from build123d import *

# Parameters (mm, degrees)
SKETCH_4_R          = 1.5
CUT_EXTRUDE_1_DEPTH = 20
SKETCH_5_R          = 1.5
CUT_EXTRUDE_2_DEPTH = 65.884590004
SKETCH3_R           = 5
SKETCH3_W           = 30
SKETCH3_H           = 42
CUT_EXTRUDE1_DEPTH  = 65.884590004
CUT_EXTRUDE2_DEPTH  = 42
CUT_EXTRUDE_3_DEPTH = 0.6


with BuildPart() as part:
    # Эскиз1 → Loft 1 section 0
    with BuildSketch(Plane(origin=(0, 0, 0), x_dir=(1, 0, 0), z_dir=(0, 1, 0))):
        with BuildLine():
            Line((-50.1, -40), (50.1, -40))
            Line((50.1, -40), (50.1, 40))
            Line((50.1, 40), (-50.1, 40))
            Line((-50.1, 40), (-50.1, -40))
        make_face()
    # Эскиз2 → Loft 1 section 1
    with BuildSketch(Plane(origin=(0, 10, 0), x_dir=(1, 0, 0), z_dir=(0, 1, 0))):
        with BuildLine():
            Line((40.1, -30), (40.1, 30))
            Line((40.1, 30), (-40.1, 30))
            Line((-40.1, 30), (-40.1, -30))
            Line((-40.1, -30), (40.1, -30))
        make_face()
    loft()

    # Эскиз4 → Вырез-Вытянуть1 (cut)
    with BuildSketch(Plane.XY.offset(40)):
        with Locations((-35.1, 5)):
            Circle(SKETCH_4_R)
        with Locations(Location((35.1, 5, 0), (0, 0, 270))):
            Circle(SKETCH_4_R)
    cut_extrude_1 = extrude(amount=-CUT_EXTRUDE_1_DEPTH, mode=Mode.SUBTRACT)

    # Зеркальное отражение1: Вырез-Вытянуть1 across plane
    add(cut_extrude_1.mirror(Plane.XY), mode=Mode.SUBTRACT)

    # Эскиз5 → Вырез-Вытянуть2 (cut, through all)
    with BuildSketch(Plane.XZ):
        with Locations(Location((-45.1, 15, 0), (0, 0, 270))):
            Circle(SKETCH_5_R)
        with Locations(Location((-45.1, -15, 0), (0, 0, 180))):
            Circle(SKETCH_5_R)
        with Locations(Location((45.1, -15, 0), (0, 0, 270))):
            Circle(SKETCH_5_R)
        with Locations((45.1, 15)):
            Circle(SKETCH_5_R)
    extrude(amount=-CUT_EXTRUDE_2_DEPTH, mode=Mode.SUBTRACT)

    # Cut-Loft1: read off the stored shape, not the designer's step
    # Cut-Loft1: loft between two sections, ruled curve by curve
    cut_loft1_from = [
        Edge.make_bspline([(-43.923484762, 2.8, 15.930490137), (-45.784465036, 2.8, 18.283520613), (-48.137495512, 2.8, 16.422540339), (-46.276515238, 2.8, 14.069509863), (-44.415534964, 2.8, 11.716479387), (-42.062504488, 2.8, 13.577459661), (-43.923484762, 2.8, 15.930490137)], [0, 0, 0, 0, 0.5, 0.5, 0.5, 1, 1, 1, 1], 3, [1, 0.333333333, 0.333333333, 1, 0.333333333, 0.333333333, 1]),
    ]
    cut_loft1_to = [
        Edge.make_bspline([(-43.881334244, 0, 18.066733405), (-50.014801053, 0, 20.504064917), (-52.452132565, 0, 14.370598107), (-46.318665756, 0, 11.933266595), (-40.185198947, 0, 9.495935083), (-37.747867435, 0, 15.629401893), (-43.881334244, 0, 18.066733405)], [0, 0, 0, 0, 0.5, 0.5, 0.5, 1, 1, 1, 1], 3, [1, 0.333333333, 0.333333333, 1, 0.333333333, 0.333333333, 1]),
    ]
    cut_loft1 = Solid(Shell([*[Face.make_surface_from_curves(cut_loft1_from[k], cut_loft1_to[k]) for k in range(1)], Face(Wire(cut_loft1_from)), Face(Wire(cut_loft1_to))]))
    add(cut_loft1, mode=Mode.SUBTRACT)

    # Mirror1: Cut-Loft1 across plane
    add(cut_loft1.mirror(Plane.XY), mode=Mode.SUBTRACT)

    # Mirror2: read off the stored shape, not the designer's step
    # Mirror2: loft between two sections, ruled curve by curve
    mirror2_from = [
        Edge.make_bspline([(43.923484762, 2.8, 15.930490137), (45.784465036, 2.8, 18.283520613), (48.137495512, 2.8, 16.422540339), (46.276515238, 2.8, 14.069509863), (44.415534964, 2.8, 11.716479387), (42.062504488, 2.8, 13.577459661), (43.923484762, 2.8, 15.930490137)], [0, 0, 0, 0, 0.5, 0.5, 0.5, 1, 1, 1, 1], 3, [1, 0.333333333, 0.333333333, 1, 0.333333333, 0.333333333, 1]),
    ]
    mirror2_to = [
        Edge.make_bspline([(43.881334244, 0, 18.066733405), (50.014801053, 0, 20.504064917), (52.452132565, 0, 14.370598107), (46.318665756, 0, 11.933266595), (40.185198947, 0, 9.495935083), (37.747867435, 0, 15.629401893), (43.881334244, 0, 18.066733405)], [0, 0, 0, 0, 0.5, 0.5, 0.5, 1, 1, 1, 1], 3, [1, 0.333333333, 0.333333333, 1, 0.333333333, 0.333333333, 1]),
    ]
    mirror2 = Solid(Shell([*[Face.make_surface_from_curves(mirror2_from[k], mirror2_to[k]) for k in range(1)], Face(Wire(mirror2_from)), Face(Wire(mirror2_to))]))
    add(mirror2, mode=Mode.SUBTRACT)

    # Mirror2 2: loft between two sections, ruled curve by curve
    mirror2_2_from = [
        Edge.make_bspline([(43.923484762, 2.8, -15.930490137), (45.784465036, 2.8, -18.283520613), (48.137495512, 2.8, -16.422540339), (46.276515238, 2.8, -14.069509863), (44.415534964, 2.8, -11.716479387), (42.062504488, 2.8, -13.577459661), (43.923484762, 2.8, -15.930490137)], [0, 0, 0, 0, 0.5, 0.5, 0.5, 1, 1, 1, 1], 3, [1, 0.333333333, 0.333333333, 1, 0.333333333, 0.333333333, 1]),
    ]
    mirror2_2_to = [
        Edge.make_bspline([(43.881334244, 0, -18.066733405), (50.014801053, 0, -20.504064917), (52.452132565, 0, -14.370598107), (46.318665756, 0, -11.933266595), (40.185198947, 0, -9.495935083), (37.747867435, 0, -15.629401893), (43.881334244, 0, -18.066733405)], [0, 0, 0, 0, 0.5, 0.5, 0.5, 1, 1, 1, 1], 3, [1, 0.333333333, 0.333333333, 1, 0.333333333, 0.333333333, 1]),
    ]
    mirror2_2 = Solid(Shell([*[Face.make_surface_from_curves(mirror2_2_from[k], mirror2_2_to[k]) for k in range(1)], Face(Wire(mirror2_2_from)), Face(Wire(mirror2_2_to))]))
    add(mirror2_2, mode=Mode.SUBTRACT)

    # Sketch3 → Cut-Extrude1 (cut, through all)
    with BuildSketch(Plane.XZ):
        with Locations(Location((-25, -12, 0), (0, 0, 270))):
            Circle(SKETCH3_R)
        with Locations((0, 2)):
            Rectangle(SKETCH3_W, SKETCH3_H)
    extrude(amount=-CUT_EXTRUDE1_DEPTH, mode=Mode.SUBTRACT)

    # Sketch4 → Cut-Extrude2 (cut)
    with BuildSketch(Plane.XY.offset(-19)):
        Polygon((-15, 8.8), (-17, 6.8), (-15, 4.8), align=None)
        Polygon((15, 4.8), (15, 8.8), (17, 6.8), align=None)
    extrude(amount=CUT_EXTRUDE2_DEPTH, mode=Mode.SUBTRACT)

    # Loft 1 2: read off the stored shape, not the designer's step
    # Loft 1 2: loft between two sections, ruled curve by curve
    loft_1_2_from = [
        Edge.make_bspline([(-23, 6.8, -18.708203932), (-14.818181818, 6.8, -16.268857048), (-14.818181818, 6.8, -7.731142952), (-23, 6.8, -5.291796068)], [0, 0, 0, 0, 1, 1, 1, 1], 3, [1, 0.523809524, 0.523809524, 1]),
        Edge.make_line((-23, 6.8, -5.291796068), (-23, 6.8, -18.708203932)),
    ]
    loft_1_2_to = [
        Edge.make_bspline([(-23, 4.8, -16.582575695), (-18.333333333, 4.8, -14.545875386), (-18.333333333, 4.8, -9.454124614), (-23, 4.8, -7.417424305)], [0, 0, 0, 0, 1, 1, 1, 1], 3, [1, 0.6, 0.6, 1]),
        Edge.make_line((-23, 4.8, -7.417424305), (-23, 4.8, -16.582575695)),
    ]
    loft_1_2 = Solid(Shell([*[Face.make_surface_from_curves(loft_1_2_from[k], loft_1_2_to[k]) for k in range(2)], Face(Wire(loft_1_2_from)), Face(Wire(loft_1_2_to))]))
    add(loft_1_2, mode=Mode.SUBTRACT)

    # Вырез-По сечениям2: read off the stored shape, not the designer's step
    # Вырез-По сечениям2: loft between two sections, ruled curve by curve
    loft_2_from = [
        Edge.make_bspline([(-27, 6.8, -5.291796068), (-35.181818182, 6.8, -7.731142952), (-35.181818182, 6.8, -16.268857048), (-27, 6.8, -18.708203932)], [0, 0, 0, 0, 1, 1, 1, 1], 3, [1, 0.523809524, 0.523809524, 1]),
        Edge.make_line((-27, 6.8, -18.708203932), (-27, 6.8, -5.291796068)),
    ]
    loft_2_to = [
        Edge.make_bspline([(-27, 4.8, -7.417424305), (-31.666666667, 4.8, -9.454124614), (-31.666666667, 4.8, -14.545875386), (-27, 4.8, -16.582575695)], [0, 0, 0, 0, 1, 1, 1, 1], 3, [1, 0.6, 0.6, 1]),
        Edge.make_line((-27, 4.8, -16.582575695), (-27, 4.8, -7.417424305)),
    ]
    loft_2 = Solid(Shell([*[Face.make_surface_from_curves(loft_2_from[k], loft_2_to[k]) for k in range(2)], Face(Wire(loft_2_from)), Face(Wire(loft_2_to))]))
    add(loft_2, mode=Mode.SUBTRACT)

    # Зеркальное отражение2: Loft 1 2, Вырез-По сечениям2 across plane
    add(loft_1_2.mirror(Plane(origin=(0, 6.8, 0), x_dir=(0, 0, 1), z_dir=(0, -1, 0))), mode=Mode.SUBTRACT)
    add(loft_2.mirror(Plane(origin=(0, 6.8, 0), x_dir=(0, 0, 1), z_dir=(0, -1, 0))), mode=Mode.SUBTRACT)

    # Эскиз8 → Вырез-Вытянуть3 (cut)
    with BuildSketch(Plane.XZ):
        Polygon((-35.1, 5), (-35.1, -25), (-5.1, -25), (-5.1, -25.5), (-4.1, -24.5), (-5.1, -23.5), (-5.1, -24), (-34.1, -24), (-34.1, 5), (-33.6, 5), (-34.6, 6), (-35.6, 5), align=None)
    extrude(amount=-CUT_EXTRUDE_3_DEPTH, mode=Mode.SUBTRACT)


solid = part.part
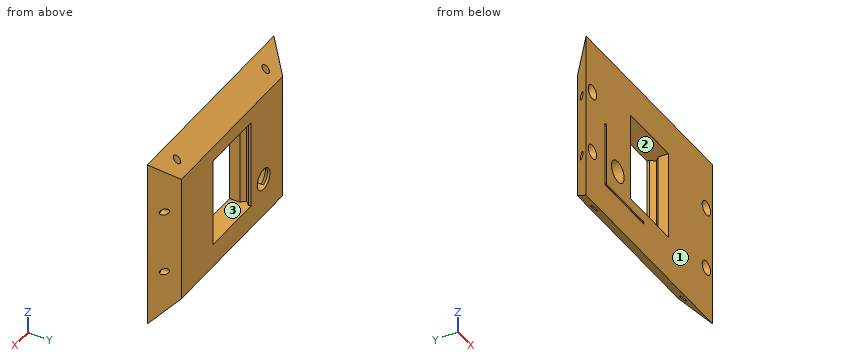
CAD build for the part. Positions are in the model's coordinates, mm. Face numbers are marked on the shaded views. Coordinates: 2 decimals unless noted, no trailing zeros. Write item = value, one per line. Start each with the question number.
Q1. Drill centre lines: L1, parallel to X at y = 5.5, z = -9; L2, parallel to X at y = 4.5, z = 15; L3, parallel to X at y = 5, z = -27.5. Where is each one in solid material? Low to high.
Q2. Flat gauge pins, fed straight in: pin 1 Ø1.5 at (x, y) = (-35, 5) entering from -Z; pin 2 Ø6 at (x, y) = (-21, 5.5) entering from -Z; pin 3 Ø2.5 at (x, z) = (45.1, -15) entering from -Y; pin 4 Ø1.1 at (y, z) = (7.5, -6.5) entering from +X. Where does each tip first touch, or does it go through?
Q3. Cut at A-A, the plane x = -45.1. Give the number of separate pieces and of enclosed holes in the cut face, then the cut area to 3 significant figures.
Q4. Pull direction X, two halves, no side cores. Call the marked faces 1, 2 and 3: pulls with the +X half, pulls with the -X half, needs draft (parallel to the pull), parting line crosses it, or undercut.
Computed:
q1.L1 = -44.6 to -29.84, -20.16 to -15.7, 15.7 to 44.6
q1.L2 = -43.6 to -15, 15 to 43.6
q1.L3 = -45.1 to -36.6, -33.6 to 33.6, 36.6 to 45.1
q2.pin_1 = -20
q2.pin_2 = -37.5
q2.pin_3 = through
q2.pin_4 = 43.15
q3.separate_pieces = 3
q3.enclosed_holes = 0
q3.area = 335 mm²
q4.face_1 = needs draft
q4.face_2 = undercut
q4.face_3 = undercut
